Could you check a few things on this model? Use its own coordinates, in mm. Round coordinates to 2 decimals unless told otherwise and drop trailing zeros. Loops run counter-clockwise (first coordinate to the right, second up) from the corner with the lowest first, then second, coordinate; pieces in that order, holes last. Notation, with made-up numbers: (74.25, 12) -> (90.25, 12) arc R29 cw to (90.25, 33) -> close; hole circle Ø3 at (52, 43.5). An arc over 180 degrees is marked (long way). One line per item, written item: value.
```python
from build123d import *

# Parameters (mm, degrees)
CYLINDER058_R     = 1.7
CYLINDER058_DEPTH = 2
CYLINDER057_R     = 1.7
CYLINDER057_DEPTH = 2
BOX020_W          = 43
BOX020_H          = 15.5
BOX020_DEPTH      = 2
FILLET007_R       = 3.24


with BuildPart() as cylinder058:
    # Cylinder058 → Cylinder058 (new body)
    with BuildSketch(Plane(origin=(24.5, 21, 23), x_dir=(1, 0, 0), z_dir=(0, 0, 1))):
        Circle(CYLINDER058_R)
    extrude(amount=CYLINDER058_DEPTH)


with BuildPart() as obj1:
    # Cylinder057 → Cylinder057 (new body)
    with BuildSketch(Plane(origin=(9.5, 21, 23), x_dir=(1, 0, 0), z_dir=(0, 0, 1))):
        Circle(CYLINDER057_R)
    extrude(amount=CYLINDER057_DEPTH)


with BuildPart() as belt_cover:
    # Box020 → Box020 (new body)
    with BuildSketch(Plane(origin=(-7, 9, 23), x_dir=(1, 0, 0), z_dir=(0, 0, 1))):
        with Locations((21.5, 7.75)):
            Rectangle(BOX020_W, BOX020_H)
    extrude(amount=BOX020_DEPTH)

    # Cut043: cut obj1
    add(obj1.part, mode=Mode.SUBTRACT)

    # Cut044: cut Cylinder058
    add(cylinder058.part, mode=Mode.SUBTRACT)

    # Fillet007
    fillet007_edges = [belt_cover.edges().sort_by_distance(p)[0] for p in [
        (-7, 9, 24),
        (36, 9, 24),
        (36, 24.5, 24),
    ]]
    fillet(fillet007_edges, radius=FILLET007_R)


solid = belt_cover.part
```
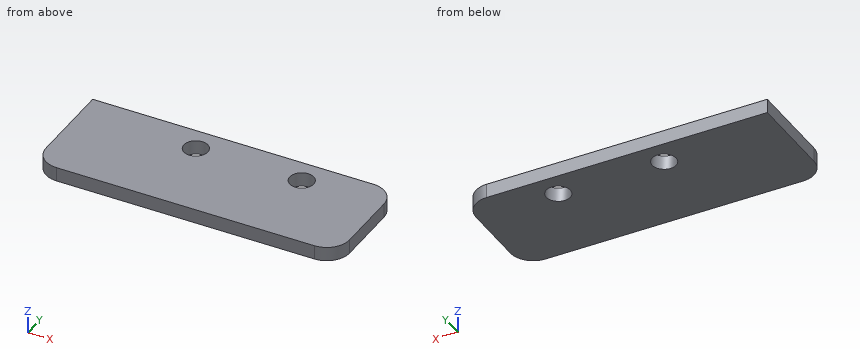
Item 1: If we section it at D-D on y = 23.5: List the corners of the cut face in (x, z) for me, plus the area to 3 significant figures.
Output:
outline: (-7, 23) -> (35.1, 23) -> (35.1, 25) -> (-7, 25) -> close
area: 84.2 mm²
Item 2: I need wall thicknesses on line 1 (Y direction, x = 9.5, z = 24.2); line 2 (X direction, y = 22.25, z = 23.95); line 3 (Y direction, x = 8, z = 24.8). Which ranges of each line are inside material? Lowest first, please. Write a range as from..to.
Output:
line 1: y = 9..19.3, 22.7..24.5
line 2: x = -7..8.35, 10.65..23.35, 25.65..35.85
line 3: y = 9..20.2, 21.8..24.5
Item 3: If we section it at A-A on z = 24.7: List the corners of the cut face in (x, y) for me, plus the area to 3 significant figures.
Output:
outline: (-7, 12.24) arc R3.24 ccw to (-3.76, 9) -> (32.76, 9) arc R3.24 ccw to (36, 12.24) -> (36, 21.26) arc R3.24 ccw to (32.76, 24.5) -> (-7, 24.5) -> close; hole circle Ø3.4 at (9.5, 21); hole circle Ø3.4 at (24.5, 21)
area: 642 mm²
Item 4: If we section it at B-B on x = 9.5: List the corners of the cut face in (y, z) for me, plus the area to 3 significant figures.
Output:
outline: (9, 23) -> (19.3, 23) -> (19.3, 25) -> (9, 25) -> close; (22.7, 23) -> (24.5, 23) -> (24.5, 25) -> (22.7, 25) -> close
area: 24.2 mm²
Item 5: Will this pin go through, and if not, where does the flat tip stop? pin 1 Ø3 at (x, y) = (9.5, 21) entering from +Z.
Output:
pin 1: passes through
Item 6: If we section it at C-C on y = 10.75: List the corners of the cut face in (x, z) for me, plus the area to 3 significant figures.
Output:
outline: (-6.64, 23) -> (35.64, 23) -> (35.64, 25) -> (-6.64, 25) -> close
area: 84.5 mm²
